CAD build for the part. Positions are in the model's coordinates, mm. A direction names the side the tool comes from. Round coordinates to 2 decimals unless told otherwise and drop trailing zeros. Loops run counter-clockwise (first coordinate to the right, second up) from the corner with the lowest first, then second, coordinate; pieces in that order, holes last.
from build123d import *

# Parameters (mm, degrees)
BOSS_EXTRUDE1_DEPTH      = 64
BOSS_EXTRUDE1_DEPTH_BACK = 12
SKETCH1_W                = 188.9125
SKETCH1_H                = 22.225
SKETCH3_W                = 60
SKETCH3_H                = 50
BOSS_EXTRUDE2_DEPTH      = 5
SKETCH4_R                = 11.43
SKETCH4_R_2              = 1.7499965
SKETCH4_R_3              = 1.75
CUT_EXTRUDE1_DEPTH       = 5
FILLET2_R                = 10
FILLET3_R                = 10
FILLET6_R                = 10
FILLET8_R                = 10
SKETCH18_W               = 5
SKETCH18_H               = 2
BOSS_EXTRUDE4_DEPTH      = 49.97124
SKETCH19_W               = 5
SKETCH19_H               = 2
BOSS_EXTRUDE5_DEPTH      = 49.971244
SKETCH26_R               = 2.413
CUT_EXTRUDE3_DEPTH       = 31.496
CHAMFER1_SIZE            = 7
CHAMFER2_SIZE            = 2
BOSS_EXTRUDE6_DEPTH      = 5
BOSS_EXTRUDE7_DEPTH      = 5
CUT_EXTRUDE2_DEPTH       = 126.162645094
CUT_EXTRUDE4_START       = 16.51
SKETCH27_R               = 2.413
CUT_EXTRUDE4_DEPTH       = 16.51


with BuildPart() as part:
    # Sketch1 → Boss-Extrude1 (new, two sides: drawn at the far end of the back side and taken through both)
    with BuildSketch(Plane(origin=(0, 0, 0), x_dir=(0, 0, -1), z_dir=(1, 0, 0)).offset(-BOSS_EXTRUDE1_DEPTH_BACK)):
        with Locations((-0.79375, -6.6675)):
            Rectangle(SKETCH1_W, SKETCH1_H)
    extrude(amount=BOSS_EXTRUDE1_DEPTH + BOSS_EXTRUDE1_DEPTH_BACK)

    # Sketch3 → Boss-Extrude2 (add)
    with BuildSketch(Plane(origin=(64, 8.866131276, 9.663552159), x_dir=(0, 0, -1), z_dir=(1, 0, 0))):
        with Locations((8.869802159, 20.550112642)):
            Rectangle(SKETCH3_W, SKETCH3_H)
    extrude(amount=-BOSS_EXTRUDE2_DEPTH)

    # Sketch4 → Cut-Extrude1 (cut)
    with BuildSketch(Plane(origin=(64, 0, 0), x_dir=(0, 0, -1), z_dir=(1, 0, 0))):
        with Locations((0, 25.6032)):
            Circle(SKETCH4_R)
        with Locations((-15.5, 41.945)):
            Circle(SKETCH4_R_2)
        with Locations((15.5, 41.945)):
            Circle(SKETCH4_R_2)
        with Locations((-15.5, 10.945)):
            Circle(SKETCH4_R_3)
        with Locations((15.5, 10.945)):
            Circle(SKETCH4_R_3)
    extrude(amount=-CUT_EXTRUDE1_DEPTH, mode=Mode.SUBTRACT)

    # Fillet2
    fillet2_edges = [part.edges().sort_by_distance(p)[0] for p in [
        (-12, -6.6675, 95.25),
    ]]
    fillet(fillet2_edges, radius=FILLET2_R)

    # Fillet3
    fillet3_edges = [part.edges().sort_by_distance(p)[0] for p in [
        (64, -6.6675, 95.25),
    ]]
    fillet(fillet3_edges, radius=FILLET3_R)

    # Fillet6
    fillet6_edges = [part.edges().sort_by_distance(p)[0] for p in [
        (-12, -6.6675, -93.6625),
    ]]
    fillet(fillet6_edges, radius=FILLET6_R)

    # Fillet8
    fillet8_edges = [part.edges().sort_by_distance(p)[0] for p in [
        (64, -6.6675, -93.6625),
    ]]
    fillet(fillet8_edges, radius=FILLET8_R)

    # Sketch18 → Boss-Extrude4 (add)
    with BuildSketch(Plane(origin=(0, 4.445, 0), x_dir=(1, 0, 0), z_dir=(0, 1, 0))):
        with Locations((61.5, -31.79375)):
            Rectangle(SKETCH18_W, SKETCH18_H)
    extrude(amount=BOSS_EXTRUDE4_DEPTH)

    # Sketch19 → Boss-Extrude5 (add)
    with BuildSketch(Plane(origin=(0, 4.445, 0), x_dir=(1, 0, 0), z_dir=(0, 1, 0))):
        with Locations((61.5, 30.20625)):
            Rectangle(SKETCH19_W, SKETCH19_H)
    extrude(amount=BOSS_EXTRUDE5_DEPTH)

    # Sketch26 → Cut-Extrude3 (cut)
    with BuildSketch(Plane.XY.offset(95.25)):
        with Locations((26, -7.78)):
            Circle(SKETCH26_R)
    extrude(amount=-CUT_EXTRUDE3_DEPTH, mode=Mode.SUBTRACT)

    # Chamfer1
    chamfer1_edges = [part.edges().sort_by_distance(p)[0] for p in [
        (61.5, 4.445, -31.20625),
        (61.5, 4.445, 32.79375),
    ]]
    chamfer(chamfer1_edges, length=CHAMFER1_SIZE)

    # Chamfer2
    chamfer2_edges = [part.edges().sort_by_distance(p)[0] for p in [
        (-12, -17.78, 0.79375),
        (26, -17.78, 95.25),
        (-9.071067812, -17.78, 92.321067812),
        (64, -17.78, 0.79375),
        (61.071067812, -17.78, 92.321067812),
        (26, -17.78, -93.6625),
        (-9.071067812, -17.78, -90.733567812),
        (61.071067812, -17.78, -90.733567812),
    ]]
    chamfer(chamfer2_edges, length=CHAMFER2_SIZE)

    # Sketch20 → Boss-Extrude6 (add)
    with BuildSketch(Plane(origin=(0, 0, -31.20625), x_dir=(-1, 0, 0), z_dir=(0, 0, -1))):
        Polygon((-59, 54.416243918), (12, 4.445), (-59, 4.445), align=None)
    extrude(amount=-BOSS_EXTRUDE6_DEPTH)

    # Sketch21 → Boss-Extrude7 (add)
    with BuildSketch(Plane.XY.offset(32.79375)):
        Polygon((59, 54.416243918), (-12, 4.445), (59, 4.445), align=None)
    extrude(amount=-BOSS_EXTRUDE7_DEPTH)

    # Sketch23 → Cut-Extrude2 (cut, through all)
    with BuildSketch(Plane(origin=(0, 4.445, 0), x_dir=(1, 0, 0), z_dir=(0, 1, 0))):
        with BuildLine():
            Line((48.76, -41.29394195), (3.24, -41.29394195))
            ThreePointArc((3.24, -41.29394195), (-0.352102448, -42.781839501), (-1.84, -46.37394195))
            Line((-1.84, -46.37394195), (-1.84, -80.01))
            ThreePointArc((-1.84, -80.01), (-0.352102448, -83.602102448), (3.24, -85.09))
            Line((3.24, -85.09), (48.76, -85.09))
            ThreePointArc((48.76, -85.09), (52.352102448, -83.602102448), (53.84, -80.01))
            Line((53.84, -80.01), (53.84, -46.37394195))
            ThreePointArc((53.84, -46.37394195), (52.352102448, -42.781839501), (48.76, -41.29394195))
        make_face()
        with BuildLine():
            Line((48.76, 83.5025), (3.24, 83.5025))
            ThreePointArc((3.24, 83.5025), (-0.352102448, 82.014602448), (-1.84, 78.4225))
            Line((-1.84, 78.4225), (-1.84, 44.78644195))
            ThreePointArc((-1.84, 44.78644195), (-0.352102448, 41.194339501), (3.24, 39.70644195))
            Line((3.24, 39.70644195), (48.76, 39.70644195))
            ThreePointArc((48.76, 39.70644195), (52.352102448, 41.194339501), (53.84, 44.78644195))
            Line((53.84, 44.78644195), (53.84, 78.4225))
            ThreePointArc((53.84, 78.4225), (52.352102448, 82.014602448), (48.76, 83.5025))
        make_face()
    extrude(amount=-CUT_EXTRUDE2_DEPTH, mode=Mode.SUBTRACT)

    # Sketch27 → Cut-Extrude4 (cut)
    with BuildSketch(Plane.XY.offset(-93.6625).offset(CUT_EXTRUDE4_START)):
        with Locations((26, -7.78)):
            Circle(SKETCH27_R)
    extrude(amount=-CUT_EXTRUDE4_DEPTH, mode=Mode.SUBTRACT)


solid = part.part
Item 1: Cut at B-B (y = 2.5). List the corners of the cut face in (x, z), plus the area to 3 significant figures.
Verdict:
outline: (-12, -83.66) arc R10 ccw to (-2, -93.66) - (54, -93.66) arc R10 ccw to (64, -83.66) - (64, 85.25) arc R10 ccw to (54, 95.25) - (-2, 95.25) arc R10 ccw to (-12, 85.25) - close; hole (-1.84, -78.42) arc R5.08 ccw to (3.24, -83.5) - (48.76, -83.5) arc R5.08 ccw to (53.84, -78.42) - (53.84, -44.79) arc R5.08 ccw to (48.76, -39.71) - (3.24, -39.71) arc R5.08 ccw to (-1.84, -44.79) - close; hole (-1.84, 46.37) arc R5.08 ccw to (3.24, 41.29) - (48.76, 41.29) arc R5.08 ccw to (53.84, 46.37) - (53.84, 80.01) arc R5.08 ccw to (48.76, 85.09) - (3.24, 85.09) arc R5.08 ccw to (-1.84, 80.01) - close
area: 9,440 mm2
Item 2: 3-axis set-ups, long thin cutter, end or side, ignore diameter. For faces 4 (the flat face through (59, 7, -34)), 5 (the flat face through (59, 6, 35)), 6 (the cylindrical face through (-0.31, -6.51, 42.74)): which of +Z, -Z, +X, -X, +Y, -Y reach the whole face in a straight line?
Verdict:
face 4: -Z, -X, +Y
face 5: +Z, -X, +Y
face 6: +Y, -Y
Item 3: Cut at A-A (z = -15.5). List the corners of the cut face in (x, y) (3 decimals).
Verdict:
outline: (-12, -15.78) - (-10, -17.78) - (62, -17.78) - (64, -15.78) - (64, 9.195) - (59, 9.195) - (59, 4.445) - (-12, 4.445) - close; (59, 12.695) - (64, 12.695) - (64, 40.195) - (59, 40.195) - close; (59, 43.695) - (64, 43.695) - (64, 54.416) - (59, 54.416) - close
Item 4: Flat gauge pins, fed straight in: P1, Ø3, axis at y = 44, z = 28, coming from the -X side; P2, Ø15, axis at x = 19.5, y = 17.5, coming from the +Z side; P3, Ø10, axis at x = 37, z = -29, coming from the +Y side; P4, Ø5.5, axis at x = 26, y = -7.78, coming from the +Z side. Where does each tip first touch, or does it go through?
Verdict:
P1: stops at x = 42.07
P2: stops at z = 32.79
P3: stops at y = 42.45
P4: stops at z = 95.25
Item 5: Mould opens along Y. For faces 1 (the flat face through (61, 54.416, -1)), 2 (the cylindrical face through (27.113, -9.921, 90.241)), 3 (the conical face through (59.97, -17.24, -89.77)) say: released by +Y, released by -Y, zero draft, split by the parting line, or undercut.
Verdict:
face 1: released by +Y
face 2: undercut
face 3: released by -Y
Item 6: Cut at C-C (x = 8). State how many separate pieces and enclosed holes the cut face has, plus the area to 3 significant figures.
Verdict:
separate pieces: 3
enclosed holes: 0
area: 2,390 mm2
Item 7: Wall check: L1, parallel to Z at x = 29.5, y = -2.5; L2, parallel to Y at x = 26, z = 90.5 (3 decimals); L3, parallel to Z at x = 17, y = 24. Give the ranges that are in metal, low to high.
Verdict:
L1: z = -93.66 to -83.5, -39.71 to 41.29, 85.09 to 95.25
L2: y = -17.78 to -10.193, -5.367 to 4.445
L3: z = -31.21 to -26.21, 27.79 to 32.79
